Input: dimensioned drawing with shaded views. Units: mm. Origin: part minimum x, y, z. Round coordinates to 2 decimals unless told otherwise and drop trailing zeros. Write each loop counter-clockwise with the first axis right and the second up, starting at its lowest first coordinate (ties: lowest second). Pieces come first, ordered by that corner, then holes. Notation, with made-up numbers: (-5.5, 10) - (16.5, 10) arc R24 cw to (16.5, 43) - close; hole circle Ø5 at (-26.75, 79.5). An arc over 180 degrees is marked (long way). Write item = value, one per line. Start each with the question number.
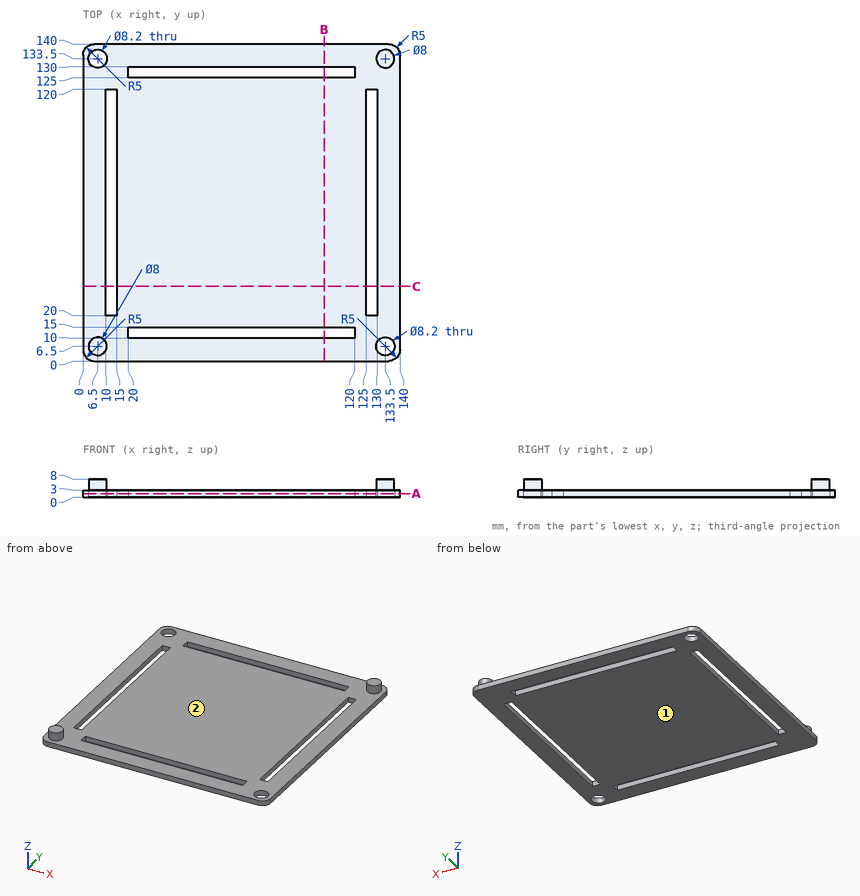
(1) Pull-direction query (Z, two-part tool) for the marked faces 1 and 2; classes: +Z half, -Z half, draft (parallel to the pull), parting line (faces both ways), or undercut.
(2) Contact query for a flat-ended pin moving along its axis: P1, Ø3, axis at x = 14.5, y = 48, coming from the +Z side. Output: stop coordinate, or through.
(3) Ray query, L1, parallel to X at y = 20.5, z = 1.25; L2, parallel to X at y = 133.5, z = 2.05. Return the intervals inside material, ascending. Write a range as from..to.
(4) Section A-A (z = 1.5). Return the cut outline in (x, y), plus the area to 3 significant figures.
(5) Section B-B (x = 106.5). Return the cut outline in (y, z).
Solution:
q1.face_1 = -Z half
q1.face_2 = +Z half
q2.P1 = 3
q3.L1 = 0..10, 15..125, 130..140
q3.L2 = 0..2.4, 10.6..140
q4.outline = (0, 5) arc R5 ccw to (5, 0) - (135, 0) arc R5 ccw to (140, 5) - (140, 135) arc R5 ccw to (135, 140) - (5, 140) arc R5 ccw to (0, 135) - close; hole circle Ø8.2 at (6.5, 133.5); hole (10, 20) - (15, 20) - (15, 120) - (10, 120) - close; hole (20, 10) - (120, 10) - (120, 15) - (20, 15) - close; hole (20, 125) - (120, 125) - (120, 130) - (20, 130) - close; hole (125, 20) - (130, 20) - (130, 120) - (125, 120) - close; hole circle Ø8.2 at (133.5, 6.5)
q4.area = 17,500 mm^2
q5.outline = (0, 0) - (10, 0) - (10, 3) - (0, 3) - close; (15, 0) - (125, 0) - (125, 3) - (15, 3) - close; (130, 0) - (140, 0) - (140, 3) - (130, 3) - close
